Verification items for this drawing (mm, ordinates from the low corner). A direction names the side the tool comes from. Coordinates: 2 decimals unless noted, no trailing zeros. Order: outer loops, then holes, each group sorted by start corner. A loop starts at its lowest first (then second) coordinate and runs counter-clockwise, first axis right, second up. Notation, with made-up numbers: (73.5, 32) -> (102.5, 32) arc R17 ccw to (102.5, 55) -> close; hole circle Ø3 at (24.5, 51.25). An arc over 180 degrees is marked (long way). Write item = value, one per line. Start each with the question number.
1. Cross-section at C-C on y = 42.5. Record the cut outline in (x, z).
2. Cross-section at D-D on x = 77. Record the cut outline in (y, z), plus the area to 3 significant figures.
3. Cross-section at A-A on x = 40. Record the cut outline in (y, z).
4. Go/stop test with flat-tipped pins: P1, Ø16.5, axis at x = 41.5, z = 45.5, coming from the +Y side; P2, Ø2, axis at y = 17, z = 27.5, coming from the -X side; P3, Ø3, axis at x = 64.5, z = 36, coming from the -Y side. Record where each tip stops, or that it passes through.
5. Thickness scan on line 1 along Z through (x, y) = (34, 128.5); line 2 along Y through (x, z) = (78.5, 49.5); line 3 along Y through (x, z) = (10, 16). Record the ranges inside material, lowest first. Write a range as from..to.
6. Cross-section at B-B on z = 13.5. Record the cut outline in (x, y).
7. Set-up check for the marked faces 1 and 2: record each of +Z, -Z, +X, -X, +Y, -Y from which the full face is reachable in a straight line by a thin tool's end or side.
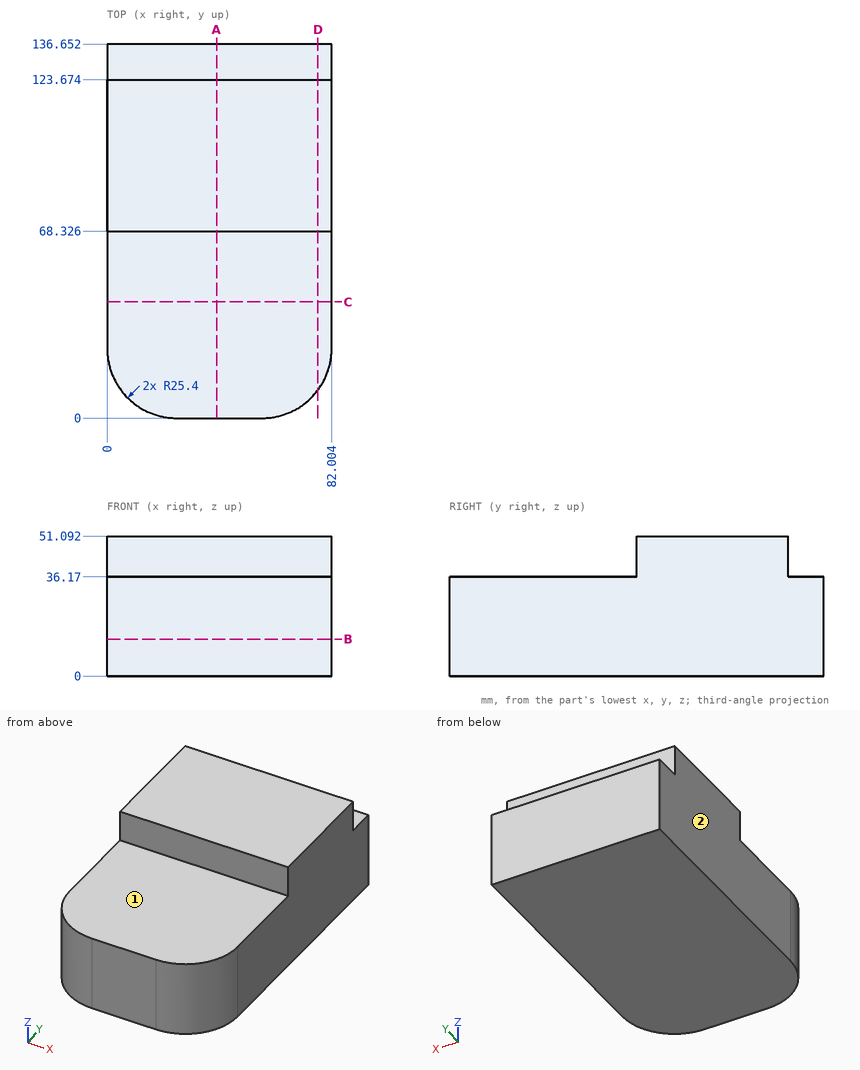
Worked out:
q1.outline = (0, 0) -> (82, 0) -> (82, 36.17) -> (0, 36.17) -> close
q2.outline = (10.26, 0) -> (136.65, 0) -> (136.65, 36.17) -> (123.67, 36.17) -> (123.67, 51.09) -> (68.33, 51.09) -> (68.33, 36.17) -> (10.26, 36.17) -> close
q2.area = 5,400 mm²
q3.outline = (0, 0) -> (136.65, 0) -> (136.65, 36.17) -> (123.67, 36.17) -> (123.67, 51.09) -> (68.33, 51.09) -> (68.33, 36.17) -> (0, 36.17) -> close
q4.P1 = 123.67
q4.P2 = 1.1
q4.P3 = 0.82
q5.line_1 = 0..36.17
q5.line_2 = 68.33..123.67
q5.line_3 = 5.2..136.65
q6.outline = (0, 25.4) arc R25.4 ccw to (25.4, 0) -> (56.6, 0) arc R25.4 ccw to (82, 25.4) -> (82, 136.65) -> (0, 136.65) -> close
q7.face_1 = +Z, +X, -X, -Y
q7.face_2 = +Z, -Z, -X, +Y, -Y
